from build123d import *

# Parameters (mm, degrees)
MEMBER_15_15_1_5_1_DEPTH = 60
SKETCH_3_R               = 1.5
CUT_EXTRUDE_1_DEPTH      = 63.299678972
SKETCH_5_R               = 1.5
CUT_EXTRUDE_2_DEPTH      = 63.299678972
SKETCH_6_R               = 1.5
CUT_EXTRUDE_3_DEPTH      = 63.299678972


with BuildPart() as part:
    # Sketch1 → Member 15 _15_ 1.5_1 (new body)
    with BuildSketch(Plane.YZ):
        Polygon((-6, -7.5), (6, -7.5), (7.5, -7.5), (7.5, -6), (7.5, 6), (7.5, 7.5), (6, 7.5), (-6, 7.5), (-7.5, 7.5), (-7.5, 6), (-7.5, -6), (-7.5, -7.5), align=None)
        Polygon((-4, -6), (4, -6), (6, -6), (6, -3.5), (6, 3.5), (6, 6), (3.5, 6), (-3.5, 6), (-5.5, 6), (-5.5, 3.5), (-5.5, -3.5), (-5.5, -6), align=None, mode=Mode.SUBTRACT)
    extrude(amount=MEMBER_15_15_1_5_1_DEPTH)

    # 草图3 → 切除-拉伸1 (cut, through all)
    with BuildSketch(Plane(origin=(0, 7.5, 0), x_dir=(1, 0, 0), z_dir=(0, 1, 0))):
        with Locations(Location((17, 0, 0), (0, 0, 270))):
            Circle(SKETCH_3_R)
        with Locations(Location((4, 0, 0), (0, 0, 270))):
            Circle(SKETCH_3_R)
    extrude(amount=-CUT_EXTRUDE_1_DEPTH, mode=Mode.SUBTRACT)

    # 草图5 → 切除-拉伸2 (cut, through all)
    with BuildSketch(Plane.XY.offset(7.5)):
        with Locations((55, 0)):
            Circle(SKETCH_5_R)
        with Locations((35, 0)):
            Circle(SKETCH_5_R)
    extrude(amount=-CUT_EXTRUDE_2_DEPTH, mode=Mode.SUBTRACT)

    # 草图6 → 切除-拉伸3 (cut, through all)
    with BuildSketch(Plane(origin=(0, 0, -7.5), x_dir=(-1, 0, 0), z_dir=(0, 0, -1))):
        with Locations((-21, 0)):
            Circle(SKETCH_6_R)
    extrude(amount=-CUT_EXTRUDE_3_DEPTH, mode=Mode.SUBTRACT)


solid = part.part
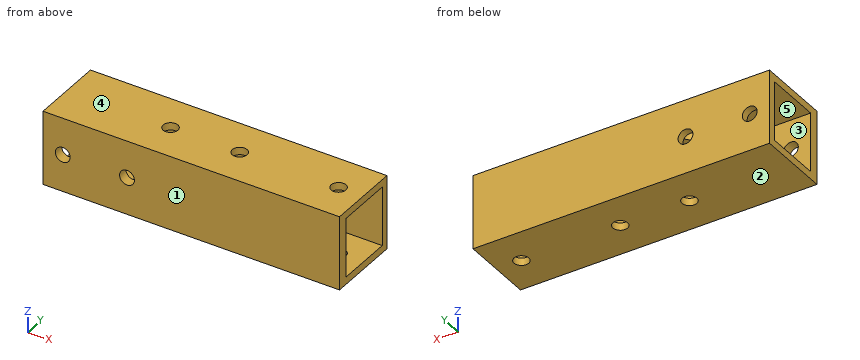
The model under review builds one solid part; all positions refer to its coordinate system, in mm. Face numbers are marked on the shaded views. A direction names the side the tool comes from. Coordinates: 2 decimals unless noted, no trailing zeros. Loops run counter-clockwise (first coordinate to the right, second up) from the corner with the lowest first, then second, coordinate; pieces in that order, holes last. Notation, with made-up numbers: M 86.5,-19.5 L 131.5,-19.5 A19 cw 131.5,-9.5 Z; hole C 39,30 d10. An arc over 180 degrees is marked long. Put each result on its own line as item: value. Start each with the question number.
Q1. Add section D-D (z = -5.25). Write out the cut boundary in (x, y).
Q2. Wall thickness on line 1 (X direction, y = -7, z = 0); line 2 (Y direction, x = 42.5, z = -5); line 3 (Y direction, x = 55, z = -7): over which ranges is each line inside the solid? List them lowest first.
Q3. Add section C-C (x = 21). Write out the cut boundary in (y, z), and give its area (3 significant figures).
Q4. For the marked faces 4 and 5, list the 3-axis set-ups (+Z, -Z, +X, -X, +Y, -Y) from which the entire face can be reached by the end or side of a thin tool; tool diameter is ignored.
Q5. Add section B-B (y = -4.75). Write out the cut boundary in (x, z), and give its area (3 significant figures).
Q6. The part is to be moulded in two halves that separate along Y. For the marked faces 1, 2 and 3, say which applies: +Y half, -Y half, draft (parallel to the pull), parting line (faces both ways), or undercut.
Q7. Add section A-A (z = 0). Write out the cut boundary in (x, y), and give its area (3 significant figures).
Q8. Clearance check with a flat-ended pin moving along its axis: pin 1 (1 mm diameter, centred on y = 3.5, z = 5, fed in from +X). State where the tip first meets the part, or that it passes through.
Answers:
1. outline: M 0,-7.5 L 60,-7.5 L 60,-5.5 L 0,-5.5 Z; M 0,6 L 60,6 L 60,7.5 L 0,7.5 Z
2. line 1: x = 0 to 2.5, 5.5 to 15.5, 18.5 to 60
2. line 2: y = -7.5 to -5.5, 6 to 7.5
2. line 3: y = -7.5 to -1.5, 1.5 to 7.5
3. outline: M -7.5,-7.5 L -1.5,-7.5 L -1.5,-6 L -5.5,-6 L -5.5,6 L -1.5,6 L -1.5,7.5 L -7.5,7.5 Z; M 1.5,-7.5 L 7.5,-7.5 L 7.5,7.5 L 1.5,7.5 L 1.5,6 L 6,6 L 6,-6 L 1.5,-6 Z
3. area: 78.0 mm^2
4. face 4: +Z, +X, -X, +Y, -Y
4. face 5: +X, -X
5. outline: M 0,-7.5 L 60,-7.5 L 60,-6 L 0,-6 Z; M 0,6 L 60,6 L 60,7.5 L 0,7.5 Z
5. area: 180 mm^2
6. face 1: -Y half
6. face 2: draft
6. face 3: undercut
7. outline: M 0,-7.5 L 2.5,-7.5 L 2.5,-5.5 L 0,-5.5 Z; M 0,6 L 2.5,6 L 2.5,7.5 L 0,7.5 Z; M 5.5,-7.5 L 15.5,-7.5 L 15.5,-5.5 L 5.5,-5.5 Z; M 5.5,6 L 15.5,6 L 15.5,7.5 L 5.5,7.5 Z; M 18.5,-7.5 L 60,-7.5 L 60,-5.5 L 18.5,-5.5 Z; M 18.5,6 L 60,6 L 60,7.5 L 18.5,7.5 Z
7. area: 189 mm^2
8. pin 1: passes through
